Read the model definition and answer for the solid it produces. Units are mm, in the model's axes. Coordinates: 2 decimals unless noted, no trailing zeros. Write each loop counter-clockwise with the first axis right and the second up, starting at its lowest first coordinate (ties: lowest second). Pieces come first, ordered by that corner, then holes.
(1) Find the intervals of material crossed by probe 1 along Y at (x, z) = (3.3, 17.5); probe 2 along Y at (x, z) = (2.85, 42); probe 3 along Z at (x, y) = (0.8, 74.5), in increasing order.
(2) Section C-C on x = 4.05 is taken. State how many separate pieces and enclosed holes the cut face has, then the cut area to 3 significant figures.
(3) Section A-A on z = 60.5 is taken. Write down the section's boundary in (x, y), then the cut area to 4 significant figures.
(4) Section B-B on y = 233 is taken. Write down the section's boundary in (x, z), then the cut area to 3 significant figures.
(5) Section D-D on y = -81 is taken. Write down the section's boundary in (x, z), then the cut area to 3 significant figures.
(6) Given pin 1 (1 mm diameter, centred on y = 130, z = 85.5, fed in from -X); pin 2 (2.5 mm diameter, centred on x = 2, z = 116.5, fed in from +Y); pin 3 (2.5 mm diameter, centred on x = 2.5, y = -38.5, fed in from -Z); pin 4 (2.5 mm diameter, centred on x = 1.5, z = 47, fed in from +Y), each flat-ended and moving along its own axis, determine where each tip first touches the part or whether it passes through.
from build123d import *

# Parameters (mm, degrees)
SKETCH_1_R      = 2
SKETCH_1_W      = 50
SKETCH_1_H      = 250
EXTRUDE_1_DEPTH = 5


with BuildPart() as part:
    # 草图1 → 凸台-拉伸1 (new body)
    with BuildSketch(Plane(origin=(0, 0, 0), x_dir=(0, 0, -1), z_dir=(1, 0, 0))):
        Polygon((-115, 195), (-115, 275), (-82.5, 275), (-82.5, 270), (-32.5, 270), (-32.5, 275), (0, 275), (0, 195), (5, 195), (5, 144.996887482), (0, 144.996887482), (0, 64.996887482), (5, 64.996887482), (5, 14.996887482), (0, 14.996887482), (0, 0), (0, -117.3), (0, -143.3), (-115, -143.3), (-115, -117.3), (-115, 0), (-115, 15), (-120, 15), (-120, 65), (-115, 65), (-115, 145), (-120, 145), (-120, 195), align=None)
        with Locations((-97.5, 145)):
            Circle(SKETCH_1_R, mode=Mode.SUBTRACT)
        with Locations((-17.5, 144.996887482)):
            Circle(SKETCH_1_R, mode=Mode.SUBTRACT)
        with Locations((-17.5, 64.996887482)):
            Circle(SKETCH_1_R, mode=Mode.SUBTRACT)
        with Locations((-97.5, 64.996887482)):
            Circle(SKETCH_1_R, mode=Mode.SUBTRACT)
        with Locations((-57.5, 120)):
            Rectangle(SKETCH_1_W, SKETCH_1_H, mode=Mode.SUBTRACT)
        with BuildLine():
            Line((-79.5, -45), (-35.5, -45))
            ThreePointArc((-35.5, -45), (-33.378679656, -45.878679656), (-32.5, -48))
            Line((-32.5, -48), (-32.5, -52))
            ThreePointArc((-32.5, -52), (-33.378679656, -54.121320344), (-35.5, -55))
            Line((-35.5, -55), (-79.5, -55))
            ThreePointArc((-79.5, -55), (-81.621320344, -54.121320344), (-82.5, -52))
            Line((-82.5, -52), (-82.5, -48))
            ThreePointArc((-82.5, -48), (-81.621320344, -45.878679656), (-79.5, -45))
        make_face(mode=Mode.SUBTRACT)
    extrude(amount=EXTRUDE_1_DEPTH)


solid = part.part
Response:
1. probe 1: y = -143.3 to 63, 67 to 143, 147 to 275
1. probe 2: y = -143.3 to -55, -45 to -5, 245 to 270
1. probe 3: z = 0 to 32.5, 82.5 to 115
2. separate pieces: 1
2. enclosed holes: 6
2. area: 35,800 mm2
3. outline: (0, -143.3) - (5, -143.3) - (5, -55) - (0, -55) - close; (0, -45) - (5, -45) - (5, -5) - (0, -5) - close; (0, 245) - (5, 245) - (5, 270) - (0, 270) - close
3. area: 766.5 mm2
4. outline: (0, 0) - (5, 0) - (5, 32.5) - (0, 32.5) - close; (0, 82.5) - (5, 82.5) - (5, 115) - (0, 115) - close
4. area: 325 mm2
5. outline: (0, 0) - (5, 0) - (5, 115) - (0, 115) - close
5. area: 575 mm2
6. pin 1: stops at x = 0
6. pin 2: stops at y = 195
6. pin 3: stops at z = 0
6. pin 4: stops at y = 270
